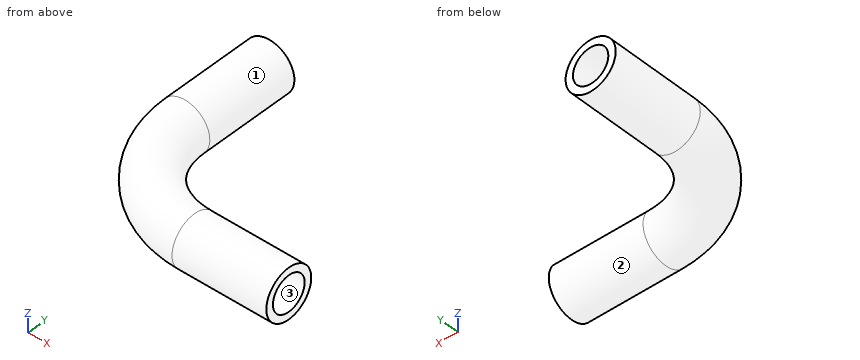
```python
from build123d import *

# Parameters (mm, degrees)
SWEEP1_PROFILE_R     = 13.49375
CUT_SWEEP1_PROFILE_R = 9.525


with BuildPart() as part:
    # Sweep1: sweep along a path in Sketch1
    with BuildLine(Plane.XY) as sweep1_path:
        Line((-50.8, 50.8), (-50.8, 0))
        ThreePointArc((-50.8, 0), (-35.921024484, -35.921024484), (0, -50.8))
        Line((0, -50.8), (50.8, -50.8))
    # Sweep1 profile (on start of the path) → Sweep1 (sweep)
    with BuildSketch(Plane(origin=(-50.8, 50.8, 0), x_dir=(0, 0, -1), z_dir=(0, -1, 0))):
        Circle(SWEEP1_PROFILE_R)
    sweep(path=sweep1_path.line)

    # Cut-Sweep1: sweep along a path in Sketch1<4>
    with BuildLine(Plane.XY) as cut_sweep1_path:
        Line((-50.8, 50.8), (-50.8, 0))
        ThreePointArc((-50.8, 0), (-35.921024484, -35.921024484), (0, -50.8))
        Line((0, -50.8), (50.8, -50.8))
    # Cut-Sweep1 profile (on start of the path) → Cut-Sweep1 (sweep, cut)
    with BuildSketch(Plane(origin=(-50.8, 50.8, 0), x_dir=(0, 0, -1), z_dir=(0, -1, 0))):
        Circle(CUT_SWEEP1_PROFILE_R)
    sweep(path=cut_sweep1_path.line, mode=Mode.SUBTRACT)


solid = part.part
```
Read the model definition and answer for the solid it produces. Units are mm, in the model's axes. Face numbers are marked on the shaded views. Give positions to 0.01 mm unless a question says otherwise; leave off trailing zeros. Write each loop counter-clockwise with the first axis right and the second up, starting at its lowest first coordinate (ties: lowest second). Pieces come first, ordered by that corner, then holes. Notation, with made-up numbers: (3.5, 85) -> (54.5, 85) arc R7 ccw to (54.5, 92) -> close; hole circle Ø11 at (10, 28). An arc over 180 degrees is marked (long way). Answer as a JSON object with one key per item and string values.
1) Section D-D on z = 6.75 is taken. Write down the section's boundary in (x, y), then the cut area to 3 significant figures.
Findings below:
{"outline": "(-62.48, 0) arc R62.48 ccw to (0, -62.48) -> (50.8, -62.48) -> (50.8, -57.52) -> (0, -57.52) arc R57.52 cw to (-57.52, 0) -> (-57.52, 50.8) -> (-62.48, 50.8) -> close; (-44.08, 0) arc R44.08 ccw to (0, -44.08) -> (50.8, -44.08) -> (50.8, -39.12) -> (0, -39.12) arc R39.12 cw to (-39.12, 0) -> (-39.12, 50.8) -> (-44.08, 50.8) -> close", "area": "1,800 mm^2"}
2) For a pull along Y with two mould halves and no side action, classify the marked faces 1, 2 and 3 as pulls with the +Y half, pulls with the -Y half, needs draft (parallel to the pull), parting line crosses it, or undercut.
Findings below:
{"face 1": "needs draft", "face 2": "parting line crosses it", "face 3": "undercut"}
3) Straight lines are drawn through the part: probe 1 along Y at (x, z) = (20, 0) (3 decimals); probe 2 along Y at (x, z) = (17, 2). For each, find the intervals that lie inside material, in ascending order. Write a range as from..to.
Findings below:
{"probe 1": "y = -64.294..-60.325, -41.275..-37.306", "probe 2": "y = -64.14..-60.11, -41.49..-37.46"}
4) Flat-ended cylindrical pins translate along their axes: pin 1 Ø10 at (x, z) = (-1.5, 3) entering from +Y; pin 2 Ø2 at (x, z) = (-25, -8.5) entering from -Y; pin 3 Ø5 at (y, z) = (-15.5, -5.5) entering from -X. Find the tip coordinate at first contact, or state that the pin passes through.
Findings below:
{"pin 1": "stops at y = -36.84", "pin 2": "stops at y = -56.87", "pin 3": "stops at x = -62.28"}
